```python
from build123d import *
from build123d.topology import SkipClean

# Parameters (mm, degrees)
CROQUIS1_W              = 70
CROQUIS1_H              = 65
EXTRUIR1_DEPTH          = 3.5
CROQUIS2_R              = 3.1
EXTRUIR2_DEPTH          = 5
EXTRUIR3_DEPTH          = 10
CROQUIS4_OUTSIDE_W      = 91.294
CROQUIS4_OUTSIDE_H      = 86.294
EXTRUIR4_DEPTH          = 10
REDONDEO1_R             = 3
EXTRUIR5_DEPTH          = 13.5
EXTRUIR6_DEPTH          = 3.5
CROQUIS7_R              = 1.6
EXTRUIR7_DEPTH          = 47.982330447
CROQUIS8_R              = 3.1
EXTRUIR8_DEPTH          = 5
CROQUIS9_W              = 0.7
CROQUIS9_H              = 10.5
EXTRUIR9_DEPTH          = 10
EXTRUIR10_DEPTH         = 63.752948337
EXTRUIR10_DEPTH_BACK    = 10
CROQUIS10_W             = 3.0625
CROQUIS10_H             = 5
CROQUIS11_W             = 54.8364
CROQUIS11_H             = 30
SALIENTE_EXTRUIR1_DEPTH = 4
CROQUIS13_W             = 7
CROQUIS13_H             = 30
SALIENTE_EXTRUIR2_DEPTH = 20
CORTAR_EXTRUIR1_DEPTH   = 8.44
CROQUIS15_W             = 22.8364
CROQUIS15_H             = 21.56
CORTAR_EXTRUIR2_DEPTH   = 8.44
CHAFL_N2_SIZE           = 3
CROQUIS16_R             = 1.5
CORTAR_EXTRUIR3_DEPTH   = 58.02817702
CHAFL_N3_SIZE           = 3


with BuildPart() as part:
    # Croquis1 → Extruir1 (new body)
    with BuildSketch(Plane(origin=(0, 0, 0), x_dir=(1, 0, 0), z_dir=(0, 1, 0))):
        Rectangle(CROQUIS1_W, CROQUIS1_H)
    extrude(amount=EXTRUIR1_DEPTH)

    # Croquis2 → Extruir2 (cut)
    with BuildSketch(Plane(origin=(0, 3.5, 0), x_dir=(1, 0, 0), z_dir=(0, 1, 0))):
        with Locations(Location((0, -17.5, 0), (0, 0, 270))):
            Circle(CROQUIS2_R)
    extrude(amount=-EXTRUIR2_DEPTH, mode=Mode.SUBTRACT)

    # Croquis3 → Extruir3 (add)
    with BuildSketch(Plane(origin=(0, 3.5, 0), x_dir=(1, 0, 0), z_dir=(0, 1, 0))):
        with BuildLine():
            Line((-34.4868, 13.5), (20.3496, 13.5))
            Line((20.3496, 13.5), (20.3496, 0))
            Line((20.3496, 0), (17.146428199, 0))
            ThreePointArc((17.146428199, 0), (22.955777517, -8.939493087), (24.418230894, -19.5))
            Line((24.418230894, -19.5), (9.287087811, -19.5))
            ThreePointArc((9.287087811, -19.5), (-3.635492607, -26.276855559), (-7.981176331, -12.347250794))
            Line((-7.981176331, -12.347250794), (-18.680510212, -1.647916913))
            ThreePointArc((-18.680510212, -1.647916913), (-17.932408832, -0.806327142), (-17.146428199, 0))
            Line((-17.146428199, 0), (-34.4868, 0))
            Line((-34.4868, 0), (-34.4868, 13.5))
        make_face()
        with BuildLine():
            Line((-32.9868, 1.5), (-12.961481397, 1.5))
            ThreePointArc((-12.961481397, 1.5), (-14.868021343, 0.048274597), (-16.613165932, -1.593940849))
            Line((-16.613165932, -1.593940849), (-5.999348286, -12.207758495))
            ThreePointArc((-5.999348286, -12.207758495), (-3.061467459, -24.89103626), (7.984359711, -18))
            Line((7.984359711, -18), (22.994564575, -18))
            ThreePointArc((22.994564575, -18), (20.451694563, -6.977253708), (12.961481397, 1.5))
            Line((12.961481397, 1.5), (18.8496, 1.5))
            Line((18.8496, 1.5), (18.8496, 12))
            Line((18.8496, 12), (-32.9868, 12))
            Line((-32.9868, 12), (-32.9868, 1.5))
        make_face(mode=Mode.SUBTRACT)
    extrude(amount=EXTRUIR3_DEPTH)

    # Croquis4 outside → Extruir4 (cut)
    with SkipClean():  # the faces are left unmerged after this step: merging them gives an invalid solid
        with BuildSketch(Plane(origin=(0, 3.5, 0), x_dir=(1, 0, 0), z_dir=(0, 1, 0))):
            Rectangle(CROQUIS4_OUTSIDE_W, CROQUIS4_OUTSIDE_H)
            with BuildLine():
                Line((-34.4868, 0), (-17.146428199, 0))
                ThreePointArc((-17.146428199, 0), (-17.932408832, -0.806327142), (-18.680510212, -1.647916913))
                Line((-18.680510212, -1.647916913), (-7.981176331, -12.347250794))
                ThreePointArc((-7.981176331, -12.347250794), (-3.635492607, -26.276855559), (9.287087811, -19.5))
                Line((9.287087811, -19.5), (24.418230894, -19.5))
                ThreePointArc((24.418230894, -19.5), (22.955777517, -8.939493087), (17.146428199, 0))
                Line((17.146428199, 0), (20.3496, 0))
                Line((20.3496, 0), (20.3496, 13.5))
                Line((20.3496, 13.5), (-34.4868, 13.5))
                Line((-34.4868, 13.5), (-34.4868, 0))
            make_face(mode=Mode.SUBTRACT)
        extrude(amount=-EXTRUIR4_DEPTH, mode=Mode.SUBTRACT)

    # Redondeo1
    redondeo1_edges = [part.edges().sort_by_distance(p)[0] for p in [
        (-7.981176331, 8.5, 12.347250794),
        (9.287087811, 8.5, 19.5),
        (-5.999348286, 8.5, 12.207758495),
        (7.984359711, 8.5, 18),
    ]]
    fillet(redondeo1_edges, radius=REDONDEO1_R)

    # Croquis5 → Extruir5 (add)
    with SkipClean():  # the faces are left unmerged after this step: merging them gives an invalid solid
        with BuildSketch(Plane.XZ):
            with BuildLine():
                Line((-18.680510212, 1.647916913), (-14.437869525, 5.8905576))
                ThreePointArc((-14.437869525, 5.8905576), (-21.723092903, 6.819250451), (-24.449770984, 0))
                Line((-24.449770984, 0), (-17.146428199, 0))
                ThreePointArc((-17.146428199, 0), (-17.932408832, 0.806327142), (-18.680510212, 1.647916913))
            make_face()
            with BuildLine():
                Line((20.3496, 0), (20.3496, -13.5))
                ThreePointArc((20.3496, -13.5), (28.665212431, 2.225567304), (24.418230894, 19.5))
                ThreePointArc((24.418230894, 19.5), (22.955777517, 8.939493087), (17.146428199, 0))
                Line((17.146428199, 0), (20.3496, 0))
            make_face()
        extrude(amount=-EXTRUIR5_DEPTH)

    # Chaflán1
    # the kernel refuses this chamfer: 5, 4.044665138 mm, written as the material it adds along each edge
    with BuildSketch(Plane(origin=(-14.437869525, 3.5, 5.8905576), x_dir=(-0.8768595348589335, 0, 0.48074666522709736), z_dir=(0, 1, 0))) as chafl_n1_piece_1:
        with BuildLine():
            Line((2.949791971, 0), (-1.211824758, 3.780414953))
            Line((-1.211824758, 3.780414953), (-1.307822013, 3.752405544))
            ThreePointArc((-1.307822013, 3.752405544), (-0.651776703, 1.876825504), (-0.095997255, -0.02800941))
            Line((-0.095997255, -0.02800941), (0.02800941, -0.095997255))
            ThreePointArc((0.02800941, -0.095997255), (1.47002525, 0.136406993), (2.931105495, -0.098238565))
            Line((2.931105495, -0.098238565), (2.949791971, 0))
        make_face()
    extrude(amount=10)
    with BuildSketch(Plane(origin=(-24.449770984, 3.5, 0), x_dir=(-0.00803680374358312, 0, 0.9999677043712897), z_dir=(0, 1, 0))) as chafl_n1_piece_2:
        with BuildLine():
            Line((2.423263449, 0), (-0.064845869, -4.38542071))
            Line((-0.064845869, -4.38542071), (-0.164842639, -4.386224391))
            ThreePointArc((-0.164842639, -4.386224391), (-0.082377051, -2.193111839), (-0.09999677, -0.00080368))
            Line((-0.09999677, -0.00080368), (0.026691621, 0.096371974))
            ThreePointArc((0.026691621, 0.096371974), (1.204598314, -0.104316531), (2.411212242, 0.099271186))
            Line((2.411212242, 0.099271186), (2.423263449, 0))
        make_face()
    extrude(amount=10)
    with BuildSketch(Plane(origin=(-24.449770984, 0, 0), x_dir=(-0.9997395779240649, 0, -0.022820524363231547), z_dir=(0, 1, 0))) as chafl_n1_piece_3:
        with BuildLine():
            Line((4.385900112, 0), (-0.035828136, 2.422998574))
            Line((-0.035828136, 2.422998574), (-0.134910293, 2.409480951))
            ThreePointArc((-0.134910293, 2.409480951), (0.08649505, 1.206008973), (-0.096756078, 0.025263837))
            Line((-0.096756078, 0.025263837), (0.002282052, -0.099973958))
            ThreePointArc((0.002282052, -0.099973958), (2.194090072, -0.04994272), (4.388182164, -0.099973958))
            Line((4.388182164, -0.099973958), (4.385900112, 0))
        make_face()
    extrude(amount=3.5)
    with BuildSketch(Plane(origin=(-14.437869525, 0, 5.8905576), x_dir=(0.7254657554746629, 0, 0.6882582637597435), z_dir=(0, 1, 0))) as chafl_n1_piece_4:
        with BuildLine():
            Line((3.96989376, 0), (-0.900434913, -2.809001538))
            Line((-0.900434913, -2.809001538), (-0.98828054, -2.761219262))
            ThreePointArc((-0.98828054, -2.761219262), (-0.318834214, -1.441501248), (-0.099965384, 0.002630967))
            Line((-0.099965384, 0.002630967), (0.002630967, 0.099965384))
            ThreePointArc((0.002630967, 0.099965384), (1.986203869, 0.047760165), (3.972524727, 0.099965384))
            Line((3.972524727, 0.099965384), (3.96989376, 0))
        make_face()
    extrude(amount=3.5)


with BuildPart() as body_2:
    # Croquis6 → Extruir6 (new body)
    with BuildSketch(Plane(origin=(0, 13.5, 0), x_dir=(1, 0, 0), z_dir=(0, 1, 0))):
        with BuildLine():
            Line((-34.4868, 13.5), (-34.4868, 0))
            Line((-34.4868, 0), (-28.661374979, 0))
            Line((-28.661374979, 0), (-24.642400208, -2.323096648))
            ThreePointArc((-24.642400208, -2.323096648), (-21.929637735, -6.692039268), (-16.829963308, -7.355409896))
            Line((-16.829963308, -7.355409896), (-11.752306982, -8.576120143))
            Line((-11.752306982, -8.576120143), (-9.515139435, -10.813287689))
            ThreePointArc((-9.515139435, -10.813287689), (-8.69974084, -12.321679102), (-8.843709432, -14.030302105))
            ThreePointArc((-8.843709432, -14.030302105), (-3.635492607, -26.276855559), (8.70689382, -21.3))
            ThreePointArc((8.70689382, -21.3), (9.813271565, -19.99001992), (11.456439237, -19.5))
            Line((11.456439237, -19.5), (24.418230894, -19.5))
            ThreePointArc((24.418230894, -19.5), (28.665212431, -2.225567304), (20.3496, 13.5))
            Line((20.3496, 13.5), (-34.4868, 13.5))
        make_face()
    extrude(amount=EXTRUIR6_DEPTH)


with BuildPart() as extruir7_tool:
    # Croquis7 → Extruir7 (new, through all)
    with BuildSketch(Plane(origin=(0, 17, 0), x_dir=(1, 0, 0), z_dir=(0, 1, 0))):
        with Locations(Location((-20, -2.5, 0), (0, 0, 270))):
            Circle(CROQUIS7_R)
        with Locations(Location((24, -2.5, 0), (0, 0, 270))):
            Circle(CROQUIS7_R)
    extrude(amount=-EXTRUIR7_DEPTH)


with BuildPart() as part_1:
    add(part.part)

    # Extruir7: cut by extruir7_tool
    add(extruir7_tool.part, mode=Mode.SUBTRACT)

    # Croquis9 → Extruir9 (cut)
    with BuildSketch(Plane(origin=(0, 13.5, 0), x_dir=(1, 0, 0), z_dir=(0, 1, 0))):
        with Locations((19.1996, 6.75)):
            Rectangle(CROQUIS9_W, CROQUIS9_H)
    extrude(amount=-EXTRUIR9_DEPTH, mode=Mode.SUBTRACT)

    # Croquis10 → Extruir10 (cut, two sides: drawn at the far end of the back side and taken through both)
    with BuildSketch(Plane.ZY.offset(-19.5496).offset(-EXTRUIR10_DEPTH_BACK)):
        with Locations((-8.9375, 8.5)):
            Rectangle(CROQUIS10_W, CROQUIS10_H)
    extrude(amount=EXTRUIR10_DEPTH + EXTRUIR10_DEPTH_BACK, mode=Mode.SUBTRACT)


with BuildPart() as body_2_1:
    add(body_2.part)

    # Extruir7: cut by extruir7_tool
    add(extruir7_tool.part, mode=Mode.SUBTRACT)

    # Croquis8 → Extruir8 (cut)
    with BuildSketch(Plane(origin=(0, 17, 0), x_dir=(1, 0, 0), z_dir=(0, 1, 0))):
        with Locations(Location((0, -17.5, 0), (0, 0, 270))):
            Circle(CROQUIS8_R)
    extrude(amount=-EXTRUIR8_DEPTH, mode=Mode.SUBTRACT)

    # Croquis11 → Saliente-Extruir1 (add)
    with BuildSketch(Plane(origin=(0, 0, -13.5), x_dir=(-1, 0, 0), z_dir=(0, 0, -1))):
        with Locations((7.0686, 32)):
            Rectangle(CROQUIS11_W, CROQUIS11_H)
    extrude(amount=-SALIENTE_EXTRUIR1_DEPTH)

    # Croquis13 → Saliente-Extruir2 (add)
    with BuildSketch(Plane.XY.offset(-9.5)):
        with Locations((-8.1504, 32)):
            Rectangle(CROQUIS13_W, CROQUIS13_H)
        with Locations((16.8496, 32)):
            Rectangle(CROQUIS13_W, CROQUIS13_H)
    extrude(amount=SALIENTE_EXTRUIR2_DEPTH)

    # Croquis14 → Cortar-Extruir1 (cut)
    with BuildSketch(Plane(origin=(0, 47, 0), x_dir=(1, 0, 0), z_dir=(0, 1, 0))):
        Polygon((20.3496, 13.5), (-34.4868, 13.5), (-34.4868, 9.5), (-11.6504, 9.5), (-11.6504, -10.5), (-4.6504, -10.5), (-4.6504, 9.5), (13.3496, 9.5), (13.3496, -10.5), (20.3496, -10.5), align=None)
    extrude(amount=-CORTAR_EXTRUIR1_DEPTH, mode=Mode.SUBTRACT)

    # Croquis15 → Cortar-Extruir2 (cut)
    with BuildSketch(Plane.XY.offset(-9.5)):
        with Locations((-23.0686, 27.78)):
            Rectangle(CROQUIS15_W, CROQUIS15_H)
    extrude(amount=-CORTAR_EXTRUIR2_DEPTH, mode=Mode.SUBTRACT)

    # Chaflán2
    chafl_n2_edges = [body_2_1.edges().sort_by_distance(p)[0] for p in [
        (-4.6504, 17, 0.5),
        (4.3496, 17, -9.5),
        (13.3496, 17, 0.5),
    ]]
    chamfer(chafl_n2_edges, length=CHAFL_N2_SIZE)

    # Croquis16 → Cortar-Extruir3 (cut, through all)
    with BuildSketch(Plane.XY.offset(10.5)):
        with Locations((-8.1504, 28.56)):
            Circle(CROQUIS16_R)
        with Locations((16.8496, 28.56)):
            Circle(CROQUIS16_R)
    extrude(amount=-CORTAR_EXTRUIR3_DEPTH, mode=Mode.SUBTRACT)

    # Chaflán3
    chafl_n3_edges = [body_2_1.edges().sort_by_distance(p)[0] for p in [
        (20.3496, 38.56, -1.5),
        (-11.6504, 38.56, -1.5),
    ]]
    chamfer(chafl_n3_edges, length=CHAFL_N3_SIZE)


solid = body_2_1.part
```
For this review, take the finished solid that the model builds, in its own axes (mm). A direction names the side the tool comes from. Round coordinates to 2 decimals unless told otherwise and drop trailing zeros. Write each loop counter-clockwise with the first axis right and the second up, starting at its lowest first coordinate (ties: lowest second). Pieces come first, ordered by that corner, then holes.
1) Mouldability with a two-part tool opening along Z and no side actions: class faces 1 (the face through (25.586, 15.274, 2.292)), 2 (the face through (-3.17, 18.52, 0.36)), 3 (the face through (-32, 15, 0)) as +Z half, -Z half, draft (parallel to the pull), parting line (faces both ways), or undercut.
Answer below:
face 1: undercut
face 2: draft
face 3: +Z half
2) Take a section at D-D on y = 18. Give the boundary of the cut face in (x, z).
Answer below:
outline: (-11.65, -13.5) - (20.35, -13.5) - (20.35, 10.5) - (11.35, 10.5) - (11.35, -7.5) - (-2.65, -7.5) - (-2.65, 10.5) - (-11.65, 10.5) - close
3) Take a section at C-C on z = 17.5. Give the boundary of the cut face in (x, y).
Answer below:
outline: (-9.5, 13.5) - (-3.1, 13.5) - (-3.1, 17) - (-9.5, 17) - close; (3.1, 13.5) - (25.67, 13.5) - (25.67, 17) - (3.1, 17) - close
4) Take a section at B-B on x = 0. Give the boundary of the cut face in (y, z), then the cut area to 3 significant figures.
Answer below:
outline: (13.5, -13.5) - (38.56, -13.5) - (38.56, -9.5) - (20, -9.5) - (17, -6.5) - (17, 14.4) - (13.5, 14.4) - close; (13.5, 20.6) - (17, 20.6) - (17, 27) - (13.5, 27) - close
area: 211 mm2
5) Take a section at A-A on y = 28.56. Give the boundary of the cut face in (x, z), then the cut area to 3 significant figures.
Answer below:
outline: (-11.65, -13.5) - (-9.65, -13.5) - (-9.65, 10.5) - (-11.65, 10.5) - close; (-6.65, -13.5) - (15.35, -13.5) - (15.35, 10.5) - (13.35, 10.5) - (13.35, -9.5) - (-4.65, -9.5) - (-4.65, 10.5) - (-6.65, 10.5) - close; (18.35, -13.5) - (20.35, -13.5) - (20.35, 10.5) - (18.35, 10.5) - close
area: 264 mm2
6) For line 1 along X through (y, z) = (34, 4.5); line 2 along X through (y, z) = (27.25, 6.5); line 3 along X through (y, z) = (15.9, 2.5), list the stretches that pass through material, from the lowest coordinate up.
Answer below:
line 1: x = -11.65 to -4.65, 13.35 to 20.35
line 2: x = -11.65 to -8.88, -7.42 to -4.65, 13.35 to 16.12, 17.58 to 20.35
line 3: x = -24.62 to -21.6, -18.4 to 22.4, 25.6 to 28.7
7) Machinability: for faces 4 (the face through (18, 15, 19.5)), 5 (the face through (-11.65, 26, -2)), 6 (the face through (-8, 26, 10.5)), 7 (the face through (4, 29, -9.5)), which of the approach directions +Z, -Z, +X, -X, +Y, -Y give a long, thin tool a straight path to every point of the face, cutting with its end or side? Answer none if there is none.
Answer below:
face 4: +Z, +X, +Y, -Y
face 5: +Z, -Z, -X, +Y
face 6: +Z, +X, -X, +Y
face 7: +Z, +Y
8) Insertion check: pin 1 Ø2 at (x, z) = (-10.5, 10) entering from -Y; pin 2 Ø2 at (y, z) = (19, 14.5) entering from +X; pin 3 Ø1.5 at (y, z) = (26, 10.5) entering from +X; pin 4 Ø9.5 at (y, z) = (26.5, 0) entering from -X. Each pin has a flat end and moves straight along its axis. Give the tip position at first contact, or say it passes through.
Answer below:
pin 1: stops at y = 13.5
pin 2: passes through
pin 3: stops at x = 20.35
pin 4: stops at x = -11.65
